Read the model definition and answer for the solid it produces. Units are mm, in the model's axes. A direction names the side the tool comes from. Coordinates: 2 decimals unless noted, no trailing zeros. Order: outer loops, then holes, each group sorted by start corner. A loop starts at its lowest first (then second) coordinate and runs counter-clockwise, first axis right, second up.
```python
from build123d import *

# Parameters (mm, degrees)
BOSS_EXTRUDE1_DEPTH = 11.8
SKETCH2_R           = 2
CUT_EXTRUDE1_DEPTH  = 12.8


with BuildPart() as part:
    # Sketch1 → Boss-Extrude1 (new body)
    with BuildSketch(Plane(origin=(0, 0, 0), x_dir=(1, 0, 0), z_dir=(0, 1, 0))):
        with BuildLine():
            Line((7.385621722, -4), (-7.385621722, -4))
            ThreePointArc((-7.385621722, -4), (-9.724157589, -4.580582618), (-11.519608146, -6.1875))
            ThreePointArc((-11.519608146, -6.1875), (-14.882843258, -7.367156742), (-17, -4.5))
            Line((-17, -4.5), (-17, 4))
            Line((-17, 4), (17, 4))
            Line((17, 4), (17, -4.5))
            ThreePointArc((17, -4.5), (14.882843258, -7.367156742), (11.519608146, -6.1875))
            ThreePointArc((11.519608146, -6.1875), (9.724157589, -4.580582618), (7.385621722, -4))
        make_face()
    extrude(amount=BOSS_EXTRUDE1_DEPTH)

    # Sketch2 → Cut-Extrude1 (cut, through all)
    with BuildSketch(Plane(origin=(0, 11.8, 0), x_dir=(1, 0, 0), z_dir=(0, 1, 0))):
        Circle(SKETCH2_R)
    extrude(amount=-CUT_EXTRUDE1_DEPTH, mode=Mode.SUBTRACT)


solid = part.part
```
1) A cutting plane is placed at D-D, the plane x = -10.5. Determine the outline of the cut face in (y, z), and give its area (3 significant figures).
A:
outline: (0, -4) - (11.8, -4) - (11.8, 5.09) - (0, 5.09) - close
area: 107 mm2
2) A cutting plane is placed at A-A, the plane y = 6.5. Determine the outline of the cut face in (x, z), and give its area (3 significant figures).
A:
outline: (-17, -4) - (17, -4) - (17, 4.5) arc R3 ccw to (11.52, 6.19) arc R5 cw to (7.39, 4) - (-7.39, 4) arc R5 cw to (-11.52, 6.19) arc R3 ccw to (-17, 4.5) - close; hole circle Ø4 at (0, 0)
area: 297 mm2
3) Determine the mould class of faces 3 (the cylindrical face through (0, 6, 2)), 4 (the cylindrical face through (9.754, 5.817, 4.597)), 5 (the flat face through (0, 11.8, 3)) for opening direction Z: pulls with the +Z half, pulls with the -Z half, needs draft (parallel to the pull), parting line crosses it, or undercut.
A:
face 3: undercut
face 4: pulls with the +Z half
face 5: needs draft
4) A cutting plane is placed at B-B, the plane x = 0. Determine the outline of the cut face in (y, z).
A:
outline: (0, -4) - (11.8, -4) - (11.8, -2) - (0, -2) - close; (0, 2) - (11.8, 2) - (11.8, 4) - (0, 4) - close
5) Flat-ended cylindrical pins translate along their axes: pin 1 Ø6 at (x, y) = (-5, 8.5) entering from +Z; pin 2 Ø3.5 at (x, z) = (0, 0) entering from +Y; pin 3 Ø6 at (x, y) = (10, 4.5) entering from +Z. Find the tip coordinate at first contact, or state that the pin passes through.
A:
pin 1: stops at z = 4.04
pin 2: passes through
pin 3: stops at z = 7.33
6) A cutting plane is placed at C-C, the plane z = 0. Determine the outline of the cut face in (x, y).
A:
outline: (-17, 0) - (-2, 0) - (-2, 11.8) - (-17, 11.8) - close; (2, 0) - (17, 0) - (17, 11.8) - (2, 11.8) - close
7) Straight lines are drawn through the part: line 1 (Z direction, x = 0, y = 6); line 2 (X direction, y = 2.5, z = 0); line 3 (Z direction, x = -3.5, y = 1). For each, find the intervals that lie inside material, in ascending order.
A:
line 1: z = -4 to -2, 2 to 4
line 2: x = -17 to -2, 2 to 17
line 3: z = -4 to 4
8) Which of the six approach directions +Z, -Z, +X, -X, +Y, -Y give full straight-line access (tool end or side, diameter ignored) to faces 1 (the cylindrical face through (-9.694, 5.817, 4.565)), 2 (the flat face through (-17, 6, 0))?
A:
face 1: +Z, +Y, -Y
face 2: +Z, -Z, -X, +Y, -Y
